Geometry: final body of the model. Coordinates: model frame, mm. Coordinates: 2 decimals unless noted, no trailing zeros. Loops run counter-clockwise (first coordinate to the right, second up) from the corner with the lowest first, then second, coordinate; pieces in that order, holes last. Notation, with made-up numbers: M 63.25,13 L 89.25,13 A18 cw 89.25,44 Z; hole C -14,2.5 d7. An arc over 180 degrees is marked long. Write item = value, one per line. Start each with the question number.
```python
from build123d import *

# Parameters (mm, degrees)
F0_R     = 4.25
F1_DEPTH = 5


with BuildPart() as f1:
    # F0 (on Front) → F1 (new body)
    with BuildSketch(Plane.XZ):
        Polygon((0, 100), (0, 0), (60, 0), (75, 15), (75, 41.457359), (73.042641, 39.5), (61.957359, 39.5), (60, 41.457359), (60, 21.213203), (53.786797, 15), (15, 15), (15, 85), (53.786797, 85), (60, 78.786797), (60, 45.7), (63.2, 42.5), (71.8, 42.5), (75, 45.7), (75, 85), (60, 100), align=None)
        with Locations((67.5, 50)):
            Circle(F0_R, mode=Mode.SUBTRACT)
    extrude(amount=F1_DEPTH)


solid = f1.part
```
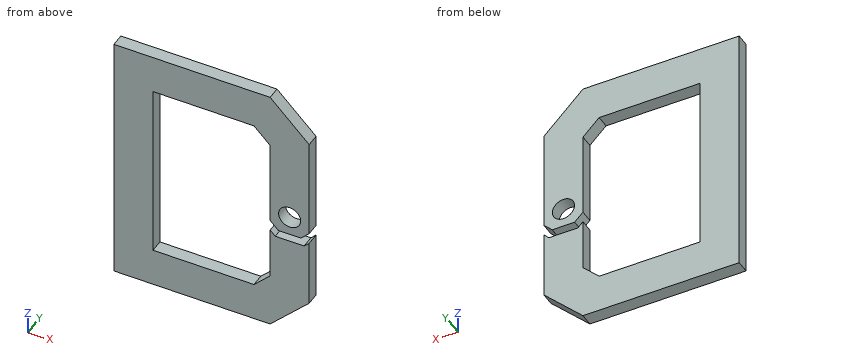
Item 1: First-contact query: pin 1 (1.5 mm diameter, centred on x = 62, y = -2.5, fed in from -Z); pin 2 (2.5 mm diameter, centred on x = 66.5, y = -2.5, fed in from +Z). Flat tips, straight axial feed; report the tip coordinate or a pass-through.
Item 2: Section query B-B (z = 32.5). Return the cut outline in (x, y), plus the area to 3 significant figures.
Item 3: Line query: line 1 (X direction, y = -0.6, z = 57); line 2 (Z direction, x = 25.5, y = -3.2); line 3 (Z direction, x = 67.5, y = -2.9). Output: solid intervals per line, ascending. Write a range as from..to.
Item 4: Section query D-D (y = -3.15). Return the cut outline in (x, z), plus the area to 3 significant figures.
Item 5: Section query A-A (x = 42). Return the cut outline in (y, z), plus the area to 3 significant figures.
Item 6: Section query C-C (x = 67.5). Return the cut outline in (y, z).
Verdict:
q1.pin_1 = 1.25
q1.pin_2 = 94.75
q2.outline = M 0,-5 L 15,-5 L 15,0 L 0,0 Z; M 60,-5 L 75,-5 L 75,0 L 60,0 Z
q2.area = 150 mm2
q3.line_1 = 0..15, 60..75
q3.line_2 = 0..15, 85..100
q3.line_3 = 7.5..39.5, 42.5..45.75, 54.25..92.5
q4.outline = M 0,0 L 60,0 L 75,15 L 75,41.46 L 73.04,39.5 L 61.96,39.5 L 60,41.46 L 60,21.21 L 53.79,15 L 15,15 L 15,85 L 53.79,85 L 60,78.79 L 60,45.7 L 63.2,42.5 L 71.8,42.5 L 75,45.7 L 75,85 L 60,100 L 0,100 Z; hole C 67.5,50 d8.5
q4.area = 4,060 mm2
q5.outline = M -5,0 L 0,0 L 0,15 L -5,15 Z; M -5,85 L 0,85 L 0,100 L -5,100 Z
q5.area = 150 mm2
q6.outline = M -5,7.5 L 0,7.5 L 0,39.5 L -5,39.5 Z; M -5,42.5 L 0,42.5 L 0,45.75 L -5,45.75 Z; M -5,54.25 L 0,54.25 L 0,92.5 L -5,92.5 Z
